Source: CAD feature listing. Evaluate the final solid. Frame: model axes, mm. Face numbers are marked on the shaded views. A direction names the side the tool comes from. Coordinates: 2 decimals unless noted, no trailing zeros. Write each loop counter-clockwise with the first axis right and the second up, starting at its lowest first coordinate (ties: lowest second). Pieces come first, ordered by that corner, then holes. Notation, with made-up numbers: (75.25, 69.25) -> (120.25, 69.25) arc R23 cw to (120.25, 100.25) -> close; hole circle Ø2 at (65, 57.25). An arc over 180 degrees is marked (long way). One line per item, written item: value. Start each with the question number.
1. Section query B-B, the plane y = -2. Output: boundary loops of the cut face in (x, z).
2. Line query: line 1 (Z direction, x = 0.5, y = -16); line 2 (Y direction, x = 0, z = 3.55); line 3 (Y direction, x = 0, z = 2.5). Output: solid intervals per line, ascending.
3. Section query D-D, the plane z = 6. Output: boundary loops of the cut face in (x, y), and give its area (3 significant figures).
4. Section query A-A, the plane z = 0. Output: boundary loops of the cut face in (x, y), and give its area (3 significant figures).
5. First-contact query: P1, Ø7, axis at x = 0.5, y = 4.5, coming from the -Z side; P2, Ø9, axis at x = -1, y = -19.5, coming from the +Z side; P3, Ø3, axis at y = -11.5, z = 1, coming from the -X side; P4, Ø4, axis at x = -3, y = 6, coming from the +Z side. Flat tips, straight axial feed; report the tip coordinate or a pass-through.
6. Mould query, pull axis Z, two halves, no side actions, for the marked faces 1, 2 and 3. Classes: released by +Z, released by -Z, zero draft, split by the parting line, or undercut.
7. Section query C-C, the plane x = 0. State how many separate pieces and enclosed holes the cut face has, and give its area (3 significant figures).
8. Access query for the marked faces 4, 5 and 6. Directions: +Z, -Z, +X, -X, +Y, -Y. A direction counts if a zero-diameter tool reaches every point of the face in a straight line with its end or side. Return the directions, or none.
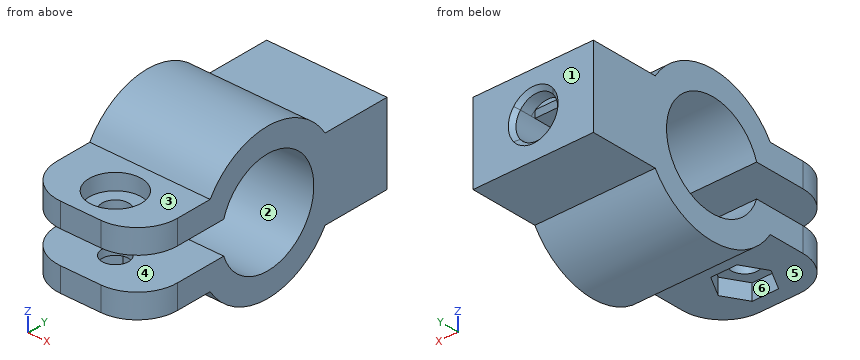
from build123d import *
from build123d import SkipClean  # not in build123d's __all__

# Parameters (mm, degrees)
F0_W           = 15
F0_H           = 10
F1_DEPTH       = 8.5
F3_DEPTH       = 7.5
F5_D           = 3.3
F5_CBORE_D     = 6.5
F5_CBORE_DEPTH = 2
F7_DEPTH       = 2
F8_R           = 5
F10_DEPTH      = 2
F11_T3_DEPTH   = 6.6704632943
F11_S4_R       = 2.6
F11_T5_DEPTH   = 5
F11_T8_DEPTH   = 6.6704632943
F11_S9_R       = 2.6
F11_T10_DEPTH  = 5
F11_T13_ANGLE  = 75.9597448897
F11_T16_ANGLE  = 75.9597448897
F11_T19_ANGLE  = 104.0402551103
F11_T22_ANGLE  = 104.0402551103


# Not quite as in the source:
# - a fillet or chamfer that OpenCascade refuses, or shapes differently, is made with other operations: its cross-section is extruded or revolved along the edge and cut away or added


with BuildPart() as f1:
    # F0 (on Front) → F1 (new body)
    with BuildSketch(Plane.XZ):
        Rectangle(F0_W, F0_H)
        with BuildLine():
            ThreePointArc((-2.0493901532, -1.6), (-2.6, 0), (-2.0493901532, 1.6))
            Line((-2.0493901532, 1.6), (2.0493901532, 1.6))
            ThreePointArc((2.0493901532, 1.6), (2.6, 0), (2.0493901532, -1.6))
            Line((2.0493901532, -1.6), (-2.0493901532, -1.6))
        make_face(mode=Mode.SUBTRACT)
    extrude(amount=-F1_DEPTH)

    # F2 (on Right) → F3 (join, symmetric)
    with BuildSketch(Plane.YZ):
        with BuildLine():
            ThreePointArc((-13.9276061789, 2), (-1.5507910996, 0), (-13.9276061789, -2))
            Line((-13.9276061789, -2), (-25.3015821993, -2))
            Line((-25.3015821993, -2), (-25.3015821993, -5))
            Line((-25.3015821993, -5), (-15.8015821993, -5))
            ThreePointArc((-15.8015821993, -5), (-7.9007910996, -9.35), (0, -5))
            Line((0, -5), (0, 5))
            ThreePointArc((0, 5), (-7.9007910996, 9.35), (-15.8015821993, 5))
            Line((-15.8015821993, 5), (-25.3015821993, 5))
            Line((-25.3015821993, 5), (-25.3015821993, 2))
            Line((-25.3015821993, 2), (-13.9276061789, 2))
        make_face()
    extrude(amount=F3_DEPTH, both=True)

    # F5 (through all)
    with Locations(Plane.XY.offset(5)):
        with Locations((0, -20.5515821993)):
            CounterBoreHole(F5_D / 2, F5_CBORE_D / 2, F5_CBORE_DEPTH)

    # F6 (on face) → F7 (cut)
    with BuildSketch(Plane(origin=(0, 0, -5), x_dir=(1, 0, 0), z_dir=(0, 0, -1))):
        Polygon((-1.6454482672, 17.7015821993), (1.6454482672, 17.7015821993), (3.2908965344, 20.5515821993), (1.6454482672, 23.4015821993), (-1.6454482672, 23.4015821993), (-3.2908965344, 20.5515821993), align=None)
    extrude(amount=-F7_DEPTH, mode=Mode.SUBTRACT)

    # F8
    f8_edges = [f1.edges().sort_by_distance(p)[0] for p in [
        (7.5, -25.301582, 3.5),
        (-7.5, -25.301582, 3.5),
        (-7.5, -25.301582, -3.5),
        (7.5, -25.301582, -3.5),
    ]]
    fillet(f8_edges, radius=F8_R)

    # F9 (on face) → F10 (cut)
    with BuildSketch(Plane(origin=(0, 8.5, 0), x_dir=(-1, 0, 0), z_dir=(0, 1, 0))):
        with BuildLine():
            Line((-2.0493901532, 1.6), (2.0493901532, 1.6))
            ThreePointArc((2.0493901532, 1.6), (0, 2.6), (-2.0493901532, 1.6))
        make_face()
        with BuildLine():
            ThreePointArc((-2.0493901532, -1.6), (0, -2.6), (2.0493901532, -1.6))
            Line((2.0493901532, -1.6), (-2.0493901532, -1.6))
        make_face()
    with SkipClean():  # cleaning this boolean's faces spoils the solid; the shape is the same uncleaned
        extrude(amount=-F10_DEPTH, mode=Mode.SUBTRACT)

    # F11: chamfer of 0.5 on 6 edges, made by hand


with BuildPart() as f11_tool1:
    # F11_s2 → F11_t3 (new body)
    with BuildSketch(Plane.YZ.offset(3.3352316472)):
        Polygon((6, 1.6), (6.5, 2.1), (6.5, 1.6), align=None)
    extrude(amount=-F11_T3_DEPTH)

    # F11_s4 → F11_t5 (intersect, symmetric)
    with BuildSketch(Plane.XZ.offset(-6.2)):
        Circle(F11_S4_R)
    extrude(amount=F11_T5_DEPTH, both=True, mode=Mode.INTERSECT)


with BuildPart() as f11_tool6:
    # F11_s7 → F11_t8 (new body)
    with BuildSketch(Plane.YZ.offset(-3.3352316472)):
        Polygon((6, -1.6), (6.5, -2.1), (6.5, -1.6), align=None)
    extrude(amount=F11_T8_DEPTH)

    # F11_s9 → F11_t10 (intersect, symmetric)
    with BuildSketch(Plane.XZ.offset(-6.2)):
        Circle(F11_S9_R)
    extrude(amount=F11_T10_DEPTH, both=True, mode=Mode.INTERSECT)


with BuildPart() as f11_tool11:
    # F11_s12 → F11_t13 (revolve)
    with BuildSketch(Plane(origin=(0, 0, 0), x_dir=(0, 1, 0), z_dir=(0.6153846154, 0, -0.788226982))):
        Polygon((8.5, -3.1), (8, -2.6), (8.5, -2.6), align=None)
    revolve(axis=Axis((0, 8.5, 0), (0, 1, 0)), revolution_arc=F11_T13_ANGLE)


with BuildPart() as f11_tool14:
    # F11_s15 → F11_t16 (revolve)
    with BuildSketch(Plane(origin=(0, 0, 0), x_dir=(0, 1, 0), z_dir=(-0.6153846154, 0, 0.788226982))):
        Polygon((8.5, -3.1), (8, -2.6), (8.5, -2.6), align=None)
    revolve(axis=Axis((0, 8.5, 0), (0, 1, 0)), revolution_arc=F11_T16_ANGLE)


with BuildPart() as f11_tool17:
    # F11_s18 → F11_t19 (revolve)
    with BuildSketch(Plane(origin=(0, 0, 0), x_dir=(0, 1, 0), z_dir=(-0.6153846154, 0, -0.788226982))):
        Polygon((8.5, -3.1), (8, -2.6), (8.5, -2.6), align=None)
    revolve(axis=Axis((0, 8.5, 0), (0, 1, 0)), revolution_arc=F11_T19_ANGLE)


with BuildPart() as f11_tool20:
    # F11_s21 → F11_t22 (revolve)
    with BuildSketch(Plane(origin=(0, 0, 0), x_dir=(0, 1, 0), z_dir=(0.6153846154, 0, 0.788226982))):
        Polygon((8.5, -3.1), (8, -2.6), (8.5, -2.6), align=None)
    revolve(axis=Axis((0, 8.5, 0), (0, 1, 0)), revolution_arc=F11_T22_ANGLE)


with BuildPart() as f1_1:
    add(f1.part, clean=False)

    # F11_t23: cut F11_tool1, F11_tool6, F11_tool11, F11_tool14, F11_tool17, F11_tool20
    add([f11_tool1.part, f11_tool6.part, f11_tool11.part, f11_tool14.part, f11_tool17.part, f11_tool20.part], mode=Mode.SUBTRACT)


solid = f1_1.part
Computed values:
1. outline: (-7.5, -7.25) -> (7.5, -7.25) -> (7.5, -2.35) -> (-7.5, -2.35) -> close; (-7.5, 2.35) -> (7.5, 2.35) -> (7.5, 7.25) -> (-7.5, 7.25) -> close
2. line 1: z = -5 to -2, 2 to 5
2. line 2: y = -25.3 to -23.8, -17.3 to -13.17, -2.64 to 8.5
2. line 3: y = -25.3 to -22.2, -18.9 to -13.74, -2.06 to 6.5
3. outline: (-7.5, -15.07) -> (7.5, -15.07) -> (7.5, -9.98) -> (-7.5, -9.98) -> close; (-7.5, -5.82) -> (7.5, -5.82) -> (7.5, -0.73) -> (-7.5, -0.73) -> close
3. area: 153 mm²
4. outline: (-7.5, -1.55) -> (7.5, -1.55) -> (7.5, 8.5) -> (3.1, 8.5) -> (2.6, 8) -> (2.6, 0) -> (-2.6, 0) -> (-2.6, 8) -> (-3.1, 8.5) -> (-7.5, 8.5) -> close
4. area: 106 mm²
5. P1: stops at z = -5
5. P2: stops at z = 6.08
5. P3: passes through
5. P4: stops at z = 5
6. face 1: zero draft
6. face 2: undercut
6. face 3: released by +Z
7. separate pieces: 3
7. enclosed holes: 0
7. area: 201 mm²
8. face 4: +X, -X, -Y
8. face 5: -Z, +X, -X, -Y
8. face 6: -Z
